Input: part model. Units: mm. Frame: model coordinates. A direction names the side the tool comes from. Round coordinates to 2 decimals unless told otherwise and drop trailing zeros. Order: outer loops, then holes, each group sorted by start corner. A loop starts at its lowest first (then second) coordinate and runs counter-clockwise, first axis right, second up. Notation, with made-up numbers: (88, 64) - (98, 64) arc R28 cw to (98, 90) - close; hole circle Ø6 at (73.25, 18). An arc over 180 degrees is marked (long way). One line per item, written item: value. Start each with the question number.
from build123d import *

# Parameters (mm, degrees)
SKETCH1_R           = 19
BOSS_EXTRUDE1_DEPTH = 2.5
BOSS_EXTRUDE2_START = 2.5
SKETCH1_3_R         = 19
SKETCH1_3_R_2       = 17.5
BOSS_EXTRUDE2_DEPTH = 17
BOSS_EXTRUDE3_START = 2.5
SKETCH1_5_R         = 2.625
SKETCH1_5_R_2       = 1.875
BOSS_EXTRUDE3_DEPTH = 17
SKETCH1_6_R         = 1.875
CUT_EXTRUDE3_DEPTH  = 34.200150602
FILLET1_R           = 2
FILLET2_R           = 2
SKETCH2_R           = 3.25
CUT_EXTRUDE5_DEPTH  = 2.5
CUT_EXTRUDE6_START  = -3
CUT_EXTRUDE6_DEPTH  = 3


with BuildPart() as part:
    # Sketch1 → Boss-Extrude1 (new body)
    with BuildSketch(Plane(origin=(0, 0, 0), x_dir=(1, 0, 0), z_dir=(0, 1, 0))):
        with Locations(Location((0, 0, 0), (0, 0, 270))):
            Circle(SKETCH1_R)
    extrude(amount=BOSS_EXTRUDE1_DEPTH)

    # Sketch1<3> → Boss-Extrude2 (add)
    with BuildSketch(Plane(origin=(0, 0, 0), x_dir=(1, 0, 0), z_dir=(0, 1, 0)).offset(BOSS_EXTRUDE2_START)):
        with Locations(Location((0, 0, 0), (0, 0, 270))):
            Circle(SKETCH1_3_R)
        with Locations(Location((0, 0, 0), (0, 0, 270))):
            Circle(SKETCH1_3_R_2, mode=Mode.SUBTRACT)
    extrude(amount=BOSS_EXTRUDE2_DEPTH)

    # Sketch1<5> → Boss-Extrude3 (add)
    with BuildSketch(Plane(origin=(0, 0, 0), x_dir=(1, 0, 0), z_dir=(0, 1, 0)).offset(BOSS_EXTRUDE3_START)):
        with Locations(Location((0, 0, 0), (0, 0, 270))):
            Circle(SKETCH1_5_R)
        with Locations(Location((0, 0, 0), (0, 0, 270))):
            Circle(SKETCH1_5_R_2, mode=Mode.SUBTRACT)
    extrude(amount=BOSS_EXTRUDE3_DEPTH)

    # Sketch1<6> → Cut-Extrude3 (cut, through all)
    with BuildSketch(Plane(origin=(0, 0, 0), x_dir=(1, 0, 0), z_dir=(0, 1, 0))):
        with Locations(Location((0, 0, 0), (0, 0, 270))):
            Circle(SKETCH1_6_R)
    extrude(amount=CUT_EXTRUDE3_DEPTH, mode=Mode.SUBTRACT)

    # Fillet1
    fillet1_edges = [part.edges().sort_by_distance(p)[0] for p in [
        (0, 0, -19),
    ]]
    fillet(fillet1_edges, radius=FILLET1_R)

    # Fillet2
    fillet2_edges = [part.edges().sort_by_distance(p)[0] for p in [
        (0, 2.5, -2.625),
        (0, 2.5, -17.5),
    ]]
    fillet(fillet2_edges, radius=FILLET2_R)

    # Sketch2 → Cut-Extrude5 (cut)
    with BuildSketch(Plane.XZ):
        with Locations(Location((0, 0, 0), (0, 0, 270))):
            Circle(SKETCH2_R)
    extrude(amount=-CUT_EXTRUDE5_DEPTH, mode=Mode.SUBTRACT)

    # Sketch3 → Cut-Extrude6 (cut)
    with BuildSketch(Plane(origin=(0, 19.5, 0), x_dir=(1, 0, 0), z_dir=(0, 1, 0)).offset(CUT_EXTRUDE6_START)):
        with BuildLine():
            Line((-4, 17.036725037), (-4, 22.5))
            Line((-4, 22.5), (-1.5, 22.5))
            Line((-1.5, 22.5), (-1.5, 17.435595774))
            ThreePointArc((-1.5, 17.435595774), (-2.757222237, 17.281427185), (-4, 17.036725037))
        make_face()
        with BuildLine():
            Line((4, 22.5), (4, 17.036725037))
            ThreePointArc((4, 17.036725037), (2.757222237, 17.281427185), (1.5, 17.435595774))
            Line((1.5, 17.435595774), (1.5, 22.5))
            Line((1.5, 22.5), (4, 22.5))
        make_face()
    cut_extrude6 = extrude(amount=CUT_EXTRUDE6_DEPTH, mode=Mode.SUBTRACT)

    # Mirror1: Cut-Extrude6 across plane
    add(cut_extrude6.mirror(Plane.XY), mode=Mode.SUBTRACT)


solid = part.part
1. Pin query (flat end, axial travel): pin 1 (1 mm diameter, centred on x = 7.5, y = 6, fed in from -Z); pin 2 (4 mm diameter, centred on x = 3, y = 2, fed in from +Z); pin 3 (1.5 mm diameter, centred on x = -9, y = 8.5, fed in from +Z). Return the tip coordinate at first contact, or that it passes through.
2. Line query: line 1 (X direction, y = 12.5, z = 0) (3 decimals); line 2 (Z direction, x = -2, y = 9.25); line 3 (Z direction, x = 1, y = 11.75). Output: solid intervals per line, ascending. Write a range as from..to.
3. Section A-A (x = 0). Return the cut outline in (y, z) (3 decimals), then the cut area to 3 significant figures.
4. Pull-direction query (X, two-part tool) for faces 1 (the face through (1.5, 18, -18)), 2 (the face through (-11.56, 10.63, -15.08)), 3 (the face through (-3, 16.5, 18)), 4 (the face through (0, 19.5, 18)); classes: released by +X, released by -X, zero draft, split by the parting line, or undercut.
5. Section B-B (y = 18). Return the cut outline in (x, z) (3 decimals), then the cut area to 3 significant figures.
6. Section C-C (z = 0). Return the cut outline in (x, y) (3 decimals).
7. Section D-D (y = 14.75). Return the cut outline in (x, z) (3 decimals).
8. Set-up query: faces 5 (the face through (-1.5, 18, 18)), 6 (the face through (-4, 18, -18)), 7 (the face through (4, 2.5, 3)). Return all of +Z, -Z, +X, -X, +Y, -Y with unobstructed straight access to the full face (end or side cutting, diameter ignored); none if empty.
Solved:
1. pin 1: stops at z = -17.66
1. pin 2: stops at z = 18.97
1. pin 3: stops at z = 17.12
2. line 1: x = -19..-17.5, -2.625..-1.875, 1.875..2.625, 17.5..19
2. line 2: z = -18.89..-17.39, -1.7..1.7, 17.39..18.89
2. line 3: z = -18.97..-17.47, -2.43..-1.59, 1.59..2.43, 17.47..18.97
3. outline: (0, -17) arc R2 ccw to (2, -19) - (19.5, -19) - (19.5, -17.5) - (4.5, -17.5) arc R2 cw to (2.5, -15.5) - (2.5, -4.625) arc R2 cw to (4.5, -2.625) - (19.5, -2.625) - (19.5, -1.875) - (2.5, -1.875) - (2.5, -3.25) - (0, -3.25) - close; (0, 3.25) - (2.5, 3.25) - (2.5, 1.875) - (19.5, 1.875) - (19.5, 2.625) - (4.5, 2.625) arc R2 cw to (2.5, 4.625) - (2.5, 15.5) arc R2 cw to (4.5, 17.5) - (19.5, 17.5) - (19.5, 19) - (2, 19) arc R2 ccw to (0, 17) - close
3. area: 157 mm²
4. face 1: undercut
4. face 2: split by the parting line
4. face 3: undercut
4. face 4: zero draft
5. outline: (-4, -18.574) - (-4, -17.037) arc R17.5 cw to (-4, 17.037) - (-4, 18.574) arc R19 ccw to start; circle Ø5.25 at (0, 0); (-1.5, -18.941) arc R19 ccw to (1.5, -18.941) - (1.5, -17.436) arc R17.5 cw to (-1.5, -17.436) - close; (-1.5, 17.436) arc R17.5 cw to (1.5, 17.436) - (1.5, 18.941) arc R19 ccw to (-1.5, 18.941) - close; (4, -18.574) arc R19 ccw to (4, 18.574) - (4, 17.037) arc R17.5 cw to (4, -17.037) - close; hole circle Ø3.75 at (0, 0)
5. area: 167 mm²
6. outline: (-19, 2) arc R2 ccw to (-17, 0) - (-3.25, 0) - (-3.25, 2.5) - (-1.875, 2.5) - (-1.875, 19.5) - (-2.625, 19.5) - (-2.625, 4.5) arc R2 cw to (-4.625, 2.5) - (-15.5, 2.5) arc R2 cw to (-17.5, 4.5) - (-17.5, 19.5) - (-19, 19.5) - close; (1.875, 2.5) - (3.25, 2.5) - (3.25, 0) - (17, 0) arc R2 ccw to (19, 2) - (19, 19.5) - (17.5, 19.5) - (17.5, 4.5) arc R2 cw to (15.5, 2.5) - (4.625, 2.5) arc R2 cw to (2.625, 4.5) - (2.625, 19.5) - (1.875, 19.5) - close
7. outline: circle Ø38 at (0, 0); circle Ø5.25 at (0, 0); hole circle Ø35 at (0, 0); hole circle Ø3.75 at (0, 0)
8. face 5: +Z, +Y
8. face 6: +Z, -Z, +Y
8. face 7: +Y
